from build123d import *

# Parameters (mm, degrees)
F0_R          = 12.7
F0_W          = 76.962
F0_H          = 22.352
F1_DEPTH      = 30.1625
F2_W          = 44.704
F2_H          = 22.3266
F3_DEPTH      = 22.353
F3_DEPTH_BACK = 22.353
F2_R          = 6.35
F4_DEPTH      = 22.353
F6_DEPTH      = 19.05
F8_DEPTH      = 19.05
F9_R          = 7.874
F10_R         = 5.08


with BuildPart() as f1:
    # F0 (on Front) → F1 (new body, symmetric)
    with BuildSketch(Plane.XZ):
        with BuildLine():
            ThreePointArc((0, -22.352), (15.8052507731, -15.8052507731), (22.352, 0))
            ThreePointArc((22.352, 0), (-15.8052507731, 15.8052507731), (0, -22.352))
        make_face()
        Circle(F0_R, mode=Mode.SUBTRACT)
        with BuildLine():
            Line((85.852, 0), (22.352, 0))
            ThreePointArc((22.352, 0), (15.8052507731, -15.8052507731), (0, -22.352))
            Line((0, -22.352), (91.8464, -22.352))
            Line((91.8464, -22.352), (85.852, 0))
        make_face()
        with Locations((155.7274, -11.176)):
            Rectangle(F0_W, F0_H)
        Polygon((117.2464, 0), (85.852, 0), (91.8464, -22.352), (117.2464, -22.352), align=None)
    extrude(amount=F1_DEPTH, both=True)

    # F2 (on face) → F3 (cut, two sides)
    with BuildSketch(Plane.XY) as f3_sk:
        Rectangle(F2_W, F2_H)
    extrude(amount=F3_DEPTH, mode=Mode.SUBTRACT)
    extrude(f3_sk.sketch, amount=-F3_DEPTH_BACK, mode=Mode.SUBTRACT)

    # F2 (on face) → F4 (cut, through all)
    with BuildSketch(Plane.XY):
        with Locations((155.3464, 7.8105)):
            Circle(F2_R)
    extrude(amount=-F4_DEPTH, mode=Mode.SUBTRACT)

    # F5 (on face) → F6 (cut)
    with BuildSketch(Plane.XZ.offset(30.1625)):
        Polygon((117.2464, 0), (85.852, 0), (91.8464, -22.352), (117.2464, -22.352), align=None)
    extrude(amount=-F6_DEPTH, mode=Mode.SUBTRACT)

    # F7 (on face) → F8 (join)
    with BuildSketch(Plane.XZ.offset(30.1625)):
        with BuildLine():
            Line((117.2464, 0), (150.0886, 0))
            Line((150.0886, 0), (150.0886, 34.798))
            Line((150.0886, 34.798), (131.0386, 34.798))
            ThreePointArc((131.0386, 34.798), (127.4644153616, 16.0823576341), (117.2464, 0))
        make_face()
    extrude(amount=-F8_DEPTH)

    # F9
    f9_edges = [f1.edges().sort_by_distance(p)[0] for p in [
        (194.2084, 0, 0),
    ]]
    fillet(f9_edges, radius=F9_R)

    # F10
    f10_edges = [f1.edges().sort_by_distance(p)[0] for p in [
        (150.0886, -20.6375, 34.798),
        (150.0886, -20.6375, 0),
        (22.352, 20.6629, 0),
        (22.352, -20.6629, 0),
    ]]
    fillet(f10_edges, radius=F10_R)


solid = f1.part
Read the model definition and answer for the solid it produces. Units are mm, in the model's axes. A direction names the side the tool comes from. Give positions to 0.01 mm unless a question says otherwise; leave off trailing zeros. Write each loop counter-clockwise with the first axis right and the second up, starting at its lowest first coordinate (ties: lowest second). Pieces come first, ordered by that corner, then holes. Notation, with made-up numbers: M 61,-34.5 L 73,-34.5 A27 cw 73,0.5 Z; hole C -20,38.25 d5. An arc over 180 degrees is marked long. One line per item, written item: value. Start each with the question number.
(1) Find section D-D (z = 20). Determine the outline of the cut face in (x, y), plus the area to 3 significant figures.
(2) Determine the mould class of faces 6 (the cylindrical face through (-2.75, -20.53, -12.4)), 7 (the flat face through (150.089, -21, 17)), 8 (the flat face through (34, -30.162, -5)) for opening direction X: pulls with the +X half, pulls with the -X half, needs draft (parallel to the pull), parting line crosses it, or undercut.
(3) Find the intervals of material crossed by line 1 (Z direction, x = 0, y = 24.5); line 2 (Y direction, x = 14, z = -5); line 3 (X direction, y = -20, z = -3), in increasing order.
(4) Flat-ended cylindrical pins translate along their axes: pin 1 Ø3 at (x, y) = (127, 12) entering from +Z; pin 2 Ø18 at (x, z) = (98.5, -10) entering from -Y; pin 3 Ø5.5 at (y, z) = (-18.5, -8.5) entering from -X. Find the tip coordinate at first contact, or state that the pin passes through.
(5) Find section C-C (x = 139.5). Determine the outline of the cut face in (y, z).
(6) A tool of negligible diameter and unlimited length cuts with its end or side. For faces 1 (the flat face through (88.8, -20.8, -11)), 2 (the cylindrical face through (-16.75, -20.8, 14.8)), 3 (the flat face through (140, -11.112, 18)), 4 (the cylindrical face through (191.841, 0.422, -2.245)), 5 (the cylindrical face through (127.56, -20.77, 16.33)), from which of +Z, -Z, +X, -X, +Y, -Y can it reach the whole face along a straight path? Write none if from no direction.
(7) Find section A-A (y = -18). Determine the outline of the cut face in (x, z).
(8) Find section B-B (y = 23). Determine the outline of the cut face in (x, z), plus the area to 3 significant figures.
Results below:
1. outline: M -9.98,-30.16 L 9.98,-30.16 L 9.98,-11.16 L -9.98,-11.16 Z; M -9.98,11.16 L 9.98,11.16 L 9.98,30.16 L -9.98,30.16 Z; M 128.83,-30.16 L 150.09,-30.16 L 150.09,-11.11 L 128.83,-11.11 Z
1. area: 1,160 mm^2
2. face 6: undercut
2. face 7: pulls with the +X half
2. face 8: needs draft
3. line 1: z = -22.35 to -12.7, 12.7 to 22.35
3. line 2: y = -30.16 to -11.16, 11.16 to 30.16
3. line 3: x = -22.15 to -12.34, 12.34 to 86.66, 117.25 to 192.52
4. pin 1: stops at z = 0
4. pin 2: stops at y = -11.11
4. pin 3: stops at x = -21.6
5. outline: M -30.16,-22.35 L 30.16,-22.35 L 30.16,0 L -11.11,0 L -11.11,34.8 L -30.16,34.8 Z
6. face 1: +Z, -Y
6. face 2: +Y, -Y
6. face 3: +Z, +X, -X, +Y
6. face 4: +Z, +X, +Y, -Y
6. face 5: +Z, +Y, -Y
7. outline: M 0,-22.35 L 91.85,-22.35 L 85.85,0 L 26.96,0 A5.08 cw 21.97,4.14 A22.35 ccw long Z; M 117.25,-22.35 L 194.21,-22.35 L 194.21,-7.87 A7.87 ccw 186.33,0 L 155.17,0 A5.08 cw 150.09,5.08 L 150.09,29.72 A5.08 ccw 145.01,34.8 L 131.04,34.8 A50.8 cw 117.25,0 Z; hole C 0,0 d25.4
8. outline: M 0,-22.35 L 194.21,-22.35 L 194.21,-7.87 A7.87 ccw 186.33,0 L 26.96,0 A5.08 cw 21.97,4.14 A22.35 ccw long Z; hole C 0,0 d25.4
8. area: 5,000 mm^2
